Check sheet for the drawn part. Datum: minimum x, y, z corner. Units: mm. A direction names the side the tool comes from. Round coordinates to 2 decimals unless told otherwise and drop trailing zeros. Loops run counter-clockwise (first coordinate to the right, second up) from the corner with the lowest first, then second, coordinate; pieces in that order, holes last.
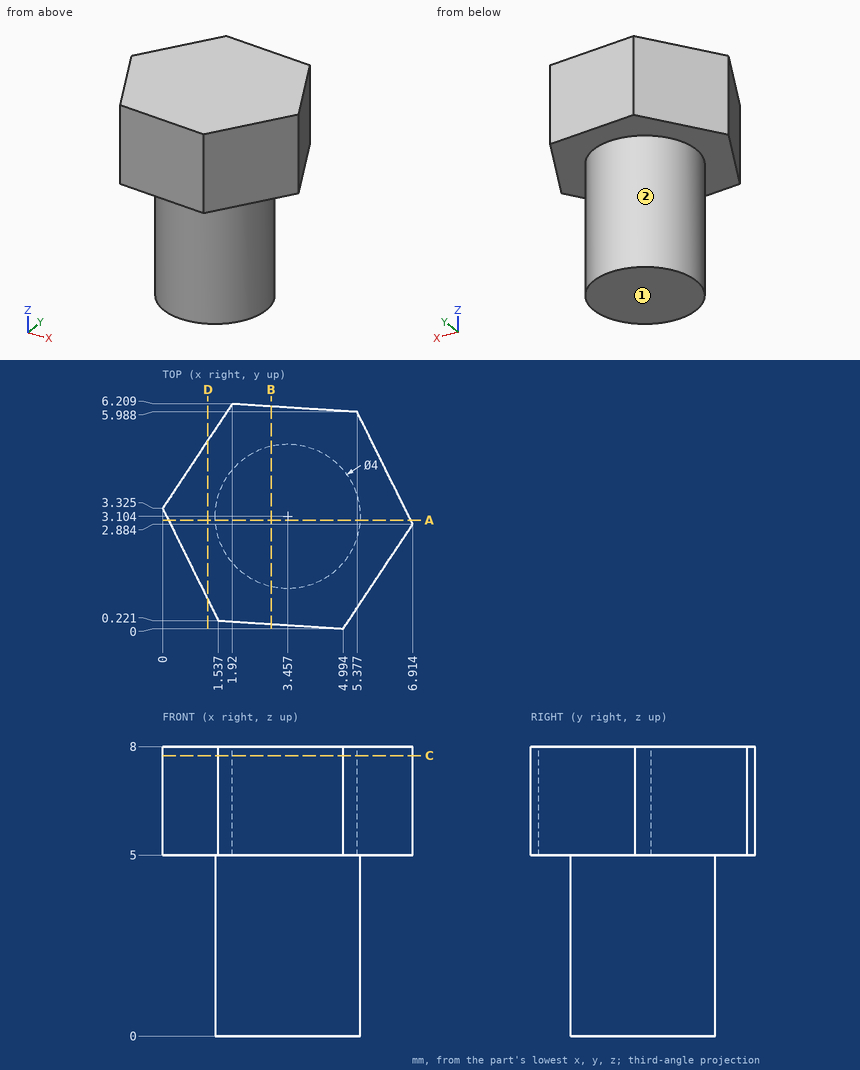
1) Sectioned sample at B-B, the plane x = 3. Record the cut outline in (y, z), then the cut area to 3 significant figures.
Report:
outline: (0.13, 5) - (1.16, 5) - (1.16, 0) - (5.05, 0) - (5.05, 5) - (6.14, 5) - (6.14, 8) - (0.13, 8) - close
area: 37.5 mm2
2) Scan lines: line 1 along Z through (x, y) = (5.5, 4.75); line 2 along Y through (x, z) = (2, 7); line 3 along Y through (x, z) = (3.5, 5.5) (1 decimal). Record each from-to range of solid material in increasing order.
Report:
line 1: z = 5 to 8
line 2: y = 0.19 to 6.2
line 3: y = 0.1 to 6.1
3) Access from +Z, -Z, +X, -X, +Y, -Y to the whole of each face (thin tool, end or side, straight path). Record for the marked faces 1 and 2.
Report:
face 1: -Z, +X, -X, +Y, -Y
face 2: -Z
4) Sectioned sample at C-C, the plane z = 7.75. Record the cut outline in (x, y) (1 decimal), then the cut area to 3 significant figures.
Report:
outline: (0, 3.3) - (1.5, 0.2) - (5, 0) - (6.9, 2.9) - (5.4, 6) - (1.9, 6.2) - close
area: 31.2 mm2
5) Sectioned sample at A-A, the plane y = 3. Record the cut outline in (x, z) (1 decimal).
Report:
outline: (0.2, 5) - (1.5, 5) - (1.5, 0) - (5.5, 0) - (5.5, 5) - (6.9, 5) - (6.9, 8) - (0.2, 8) - close
6) Sectioned sample at D-D, the plane x = 1.25. Record the cut outline in (y, z), then the cut area to 3 significant figures.
Report:
outline: (0.8, 5) - (5.2, 5) - (5.2, 8) - (0.8, 8) - close
area: 13.2 mm2
7) Gauge pin test, flat ends, axial feed: pin 1 (3 mm diameter, centred on x = 4.5, z = 4.5, fed in from +Y); pin 2 (2 mm diameter, centred on y = 2, z = 6, fed in from -X); pin 3 (1 mm diameter, centred on x = 4, z = 2, fed in from +Y). Record the tip position at first contact, or that the pin passes through.
Report:
pin 1: stops at y = 6.13
pin 2: stops at x = 0.16
pin 3: stops at y = 5.1
